from build123d import *

# Parameters (mm, degrees)
REVOLVE2_ANGLE     = 180
SKETCH13_W         = 3
SKETCH13_H         = 1
CUT_EXTRUDE1_DEPTH = 5


with BuildPart() as part:
    # Sketch2 → Revolve1 (revolve)
    with BuildSketch(Plane(origin=(0, 0, 0), x_dir=(1, 0, 0), z_dir=(0, 1, 0)), mode=Mode.PRIVATE) as revolve1_sk:
        Polygon((0, 0), (2, 0), (0, -15), align=None)
    revolve(revolve1_sk.sketch.rotate(Axis((0, 0, 15), (0, 0, -1)), 180), axis=Axis((0, 0, 15), (0, 0, -1)))

    # Sketch12 → Revolve2 (revolve)
    with BuildSketch(Plane.XY):
        with BuildLine():
            Line((0, 2.75), (0, -2.75))
            ThreePointArc((0, -2.75), (-2.75, 0), (0, 2.75))
        make_face()
    revolve(axis=Axis((0, 2.75, 0), (0, -1, 0)), revolution_arc=REVOLVE2_ANGLE)

    # Sketch13 → Cut-Extrude1 (cut, symmetric)
    with BuildSketch(Plane(origin=(0, 0, 0), x_dir=(0, 0, -1), z_dir=(1, 0, 0))):
        with Locations((2.75, 0)):
            Rectangle(SKETCH13_W, SKETCH13_H)
    extrude(amount=CUT_EXTRUDE1_DEPTH, both=True, mode=Mode.SUBTRACT)


solid = part.part
Build history of the part. All positions in model axes, mm. Round coordinates to 2 decimals unless told otherwise and drop trailing zeros. Write each loop counter-clockwise with the first axis right and the second up, starting at its lowest first coordinate (ties: lowest second). Pieces come first, ordered by that corner, then holes. Notation, with made-up numbers: M -3.75,27.5 L 11.25,27.5 A29 ccw 11.25,56.5 Z; hole C -22,20.25 d4. An arc over 180 degrees is marked long. Use CSV: the item, a comma, the result in double quotes.
1. Two-plate mould, pull along Y, no slides. Class faces 1 (the face through (-0.94, 0.3, 7.6)), 2 (the face through (0, -0.5, -2)), 3 (the face through (0, 0, -1.25)), 4 (the face through (-1, -2, 0)): +Y half, -Y half, draft (parallel to the pull), parting line (faces both ways), or undercut.
Reply:
face 1,"parting line"
face 2,"undercut"
face 3,"undercut"
face 4,"draft"
2. Wall check: probe 1 along Z at (x, y) = (0.6, -2.1); probe 2 along X at (y, z) = (-0.9, -0.5); probe 3 along X at (y, z) = (-1.6, -0.5). Give the ranges that are in metal, low to high. Write a range as from..to.
Reply:
probe 1,"z = -1.67..0"
probe 2,"x = -2.55..2.55"
probe 3,"x = -2.18..2.18"
3. Flat gauge pins, fed straight in: pin 1 (3 mm diameter, centred on x = -1, z = 8.5, fed in from +Y); pin 2 (1.2 mm diameter, centred on x = 0, z = -2.5, fed in from +Y); pin 3 (0.5 mm diameter, centred on x = -1, y = 0, fed in from -Z). Where does each tip first touch, or does it go through?
Reply:
pin 1,"stops at y = 1.02"
pin 2,"stops at y = 1.99"
pin 3,"stops at z = -1.25"
4. Saw through at B-B (z = 1). Give the cut face in (x, y).
Reply:
outline,"C 0,0 d3.73"
5. Saw through at C-C (z = 9.25). Give the cut face in (x, y), plus the area to 3 significant figures.
Reply:
outline,"C 0,0 d1.53"
area,"1.85 mm²"
6. Saw through at A-A (x = -2.2). Give the cut face in (y, z), plus the area to 3 significant figures.
Reply:
outline,"M -1.65,0 A1.65 ccw -0.5,-1.57 L -0.5,-1.25 L 0.5,-1.25 L 0.5,-1.57 A1.65 ccw 1.65,0 Z"
area,"3.90 mm²"
